from build123d import *

# Parameters (mm, degrees)
SKETCH2_W                     = 120
SKETCH2_H                     = 8
BOSS_EXTRUDE1_DEPTH           = 12
LPATTERN1_COUNT               = 5
LPATTERN1_PITCH               = 24.25
SKETCH4_R                     = 2
BOSS_EXTRUDE2_DEPTH           = 4
BOSS_EXTRUDE2_DRAFT           = 1
BOSS_EXTRUDE2_PROFILE_2_DEPTH = 4
BOSS_EXTRUDE2_PROFILE_2_DRAFT = 1


with BuildPart() as part:
    # Sketch2 → Boss-Extrude1 (new body)
    with BuildSketch(Plane.XY):
        with Locations((60, 4)):
            Rectangle(SKETCH2_W, SKETCH2_H)
    extrude(amount=-BOSS_EXTRUDE1_DEPTH)

    # Sketch3 → Cut-Revolve1 (revolve, cut)
    with BuildSketch(Plane.XY):
        Polygon((8.5, 3), (9.4, 3), (9.4, 5), (2, 5), (2, 6), (11.5, 6), (11.5, 0), (9.4, 0), align=None)
    cut_revolve1 = revolve(axis=Axis((11.5, 6, 0), (0, -1, 0)), mode=Mode.SUBTRACT)

    # LPattern1: Cut-Revolve1 ×5
    with Locations(*[(i * LPATTERN1_PITCH, 0, 0) for i in range(1, LPATTERN1_COUNT)]):
        add(cut_revolve1, mode=Mode.SUBTRACT)


with BuildPart() as boss_extrude2_tool:
    # Sketch4 → Boss-Extrude2 (with draft: the straight prism first)
    with BuildSketch(Plane.XY):
        with Locations((23.5, 3)):
            Circle(SKETCH4_R)
    extrude(amount=BOSS_EXTRUDE2_DEPTH)
    # Boss-Extrude2: the draft: its side faces are tilted about the plane it starts from
    boss_extrude2_sides = [boss_extrude2_tool.faces().sort_by_distance(p)[0] for p in [
        (21.5, 3, 2),
    ]]
    draft(boss_extrude2_sides, Plane.XY, BOSS_EXTRUDE2_DRAFT)


with BuildPart() as part_1:
    add(part.part)

    # Boss-Extrude2: add boss_extrude2_tool
    add(boss_extrude2_tool.part)


with BuildPart() as boss_extrude2_profile_2_tool:
    # Sketch4 → Boss-Extrude2 profile 2 (with draft: the straight prism first)
    with BuildSketch(Plane.XY):
        with Locations((96.5, 3)):
            Circle(SKETCH4_R)
    extrude(amount=BOSS_EXTRUDE2_PROFILE_2_DEPTH)
    # Boss-Extrude2 profile 2: the draft: its side faces are tilted about the plane it starts from
    boss_extrude2_profile_2_sides = [boss_extrude2_profile_2_tool.faces().sort_by_distance(p)[0] for p in [
        (94.5, 3, 2),
    ]]
    draft(boss_extrude2_profile_2_sides, Plane.XY, BOSS_EXTRUDE2_PROFILE_2_DRAFT)


with BuildPart() as part_2:
    add(part_1.part)

    # Boss-Extrude2 profile 2: add boss_extrude2_profile_2_tool
    add(boss_extrude2_profile_2_tool.part)


solid = part_2.part
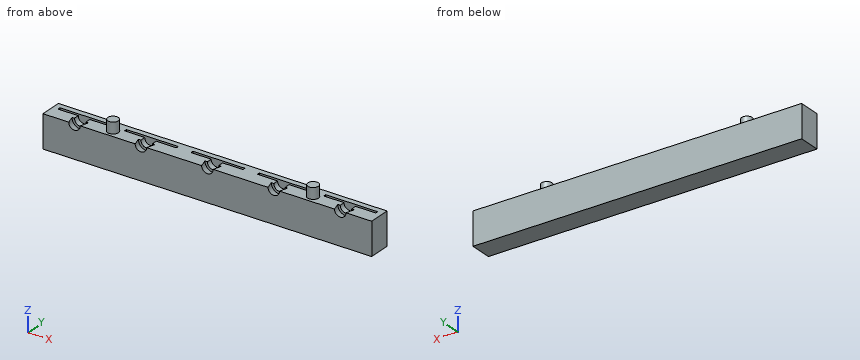
Model file for the job. Use its own axes, mm. Round coordinates to 2 decimals unless told otherwise and drop trailing zeros. Loops run counter-clockwise (first coordinate to the right, second up) from the corner with the lowest first, then second, coordinate; pieces in that order, holes last. Notation, with made-up numbers: (-10, 87.25) -> (13, 87.25) arc R21 cw to (13, 117.25) -> close; hole circle Ø8 at (86, 76.25). An arc over 180 degrees is marked (long way). Answer as CSV lines item,"result". Start each with the question number.
1) Slice it at B-B (x = 108.5). List the corners of the cut face in (y, z), plus the area to 4 significant figures.
2) Slice it at C-C (x = 53.5). List the corners of the cut face in (y, z), plus the area to 3 significant figures.
3) Slice it at D-D (z = 2). List the corners of the cut face in (x, y), plus the area to 3 significant figures.
4) Probe line 1 along Y through (x, z) = (33, -4); line 2 along X through (y, z) = (5.5, -2.5); line 3 along X through (y, z) = (5.25, -7.75). List the from-to ranges inside material, lowest first.
5) Slice it at A-A (z = -5.75). List the corners of the cut face in (x, y), plus the area to 3 significant figures.
6) Pin check, flat tips, straight feed: P1, Ø2, axis at x = 41, y = 5, coming from the +Z side; P2, Ø0.9, axis at x = 108, z = -1.5, coming from the -Y side. Stop position of each tip, or through.
Filled in:
1,outline,"(0, -12) -> (8, -12) -> (8, 0) -> (6, 0) -> (6, -9.5) -> (5, -9.5) -> (5, -2.1) -> (3, -2.1) -> (3, -3) -> (0, -2.1) -> close"
1,area,"74.65 mm2"
2,outline,"(0, -12) -> (8, -12) -> (8, 0) -> (6, 0) -> (6, -6.93) -> (5, -6.93) -> (5, 0) -> (0, 0) -> close"
2,area,"89.1 mm2"
3,outline,"circle Ø3.93 at (23.5, 3); circle Ø3.93 at (96.5, 3)"
3,area,"24.3 mm2"
4,line 1,"y = 0 to 5, 6 to 8"
4,line 2,"x = 0 to 2.33, 20.67 to 26.58, 44.92 to 50.83, 69.17 to 75.08, 93.42 to 99.33, 117.67 to 120"
4,line 3,"x = 0 to 6.01, 16.99 to 30.26, 41.24 to 54.51, 65.49 to 78.76, 89.74 to 103.01, 113.99 to 120"
5,outline,"(0, 0) -> (120, 0) -> (120, 8) -> (0, 8) -> close; hole (3.94, 5) -> (19.06, 5) -> (19.06, 6) -> (3.94, 6) -> close; hole (28.19, 5) -> (43.31, 5) -> (43.31, 6) -> (28.19, 6) -> close; hole (52.44, 5) -> (67.56, 5) -> (67.56, 6) -> (52.44, 6) -> close; hole (76.69, 5) -> (91.81, 5) -> (91.81, 6) -> (76.69, 6) -> close; hole (100.94, 5) -> (116.06, 5) -> (116.06, 6) -> (100.94, 6) -> close"
5,area,"884 mm2"
6,P1,"stops at z = 0"
6,P2,"stops at y = 6"
